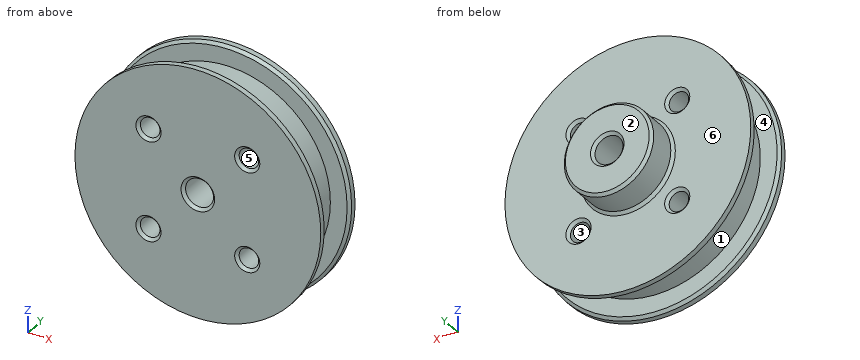
from build123d import *

# Parameters (mm, degrees)
F0_R      = 22
F1_DEPTH  = 5
F2_R      = 30.4296764291
F2_R_2    = 18.5
F3_DEPTH  = 3.5
F4_R      = 8
F5_DEPTH  = 6
F6_R      = 2.5
F7_DEPTH  = 16.001
F8_SIZE   = 0.5
F9_R      = 1.75
F10_DEPTH = 10.001
F11_SIZE  = 0.5


with BuildPart() as f1:
    # F0 (on Front) → F1 (new body, symmetric)
    with BuildSketch(Plane.XZ):
        Circle(F0_R)
    extrude(amount=F1_DEPTH, both=True)

    # F2 (on Front) → F3 (cut, symmetric)
    with BuildSketch(Plane.XZ):
        Circle(F2_R)
        Circle(F2_R_2, mode=Mode.SUBTRACT)
    extrude(amount=F3_DEPTH, both=True, mode=Mode.SUBTRACT)

    # F4 (on face) → F5 (join)
    with BuildSketch(Plane(origin=(0, 5, 0), x_dir=(-1, 0, 0), z_dir=(0, 1, 0))):
        Circle(F4_R)
    extrude(amount=F5_DEPTH)

    # F6 (on face) → F7 (cut, through all)
    with BuildSketch(Plane(origin=(0, 11, 0), x_dir=(-1, 0, 0), z_dir=(0, 1, 0))):
        Circle(F6_R)
    extrude(amount=-F7_DEPTH, mode=Mode.SUBTRACT)

    # F8
    f8_edges = [f1.edges().sort_by_distance(p)[0] for p in [
        (8, 11, 0),
        (2.5, 11, 0),
        (8, 5, 0),
        (-22, 3.5, 0),
        (-22, -3.5, 0),
        (2.5, -5, 0),
    ]]
    chamfer(f8_edges, length=F8_SIZE)

    # F9 (on face) → F10 (cut, through all)
    with BuildSketch(Plane(origin=(0, 5, 0), x_dir=(-1, 0, 0), z_dir=(0, 1, 0))):
        with Locations((-8.8388347648, 8.8388347648)):
            Circle(F9_R)
        with Locations((-8.8388347648, -8.8388347648)):
            Circle(F9_R)
        with Locations((8.8388347648, -8.8388347648)):
            Circle(F9_R)
        with Locations((8.8388347648, 8.8388347648)):
            Circle(F9_R)
    extrude(amount=-F10_DEPTH, mode=Mode.SUBTRACT)

    # F11
    f11_edges = [f1.edges().sort_by_distance(p)[0] for p in [
        (-7.088835, -5, 8.838835),
        (-7.088835, -5, -8.838835),
        (10.588835, -5, -8.838835),
        (10.588835, -5, 8.838835),
        (10.588835, 5, 8.838835),
        (-7.088835, 5, 8.838835),
        (-7.088835, 5, -8.838835),
        (10.588835, 5, -8.838835),
    ]]
    chamfer(f11_edges, length=F11_SIZE)


solid = f1.part
Design review of the part built by this model. Coordinates are the model's own, in mm. Face numbers are marked on the shaded views. A direction names the side the tool comes from. Coordinates: 2 decimals unless noted, no trailing zeros. Loops run counter-clockwise (first coordinate to the right, second up) from the corner with the lowest first, then second, coordinate; pieces in that order, holes last. Notation, with made-up numbers: M 20,-1 L 33,-1 A17 ccw 33,20 Z; hole C 17.25,9 d10. An arc over 180 degrees is marked long. Answer as CSV lines item,"result".
Item 1: Add section D-D on y = 8.5. State the section outline as (x, z) points, plus the area to 3 significant figures.
Answer list:
outline,"C 0,0 d16; hole C 0,0 d5"
area,"181 mm²"
Item 2: For P1, Ø6, axis at x = -1.5, y = 9, coming from the -Z side; P2, Ø5, axis at x = 12, y = 6, coming from the -Z side; P3, Ø1, axis at x = 16, y = 1, coming from the -Z side, all flat-tipped, find the tip position at first contact; note any pin that passes through.
Answer list:
P1,"z = -8"
P2,"z = -19.74"
P3,"z = -10.1"
Item 3: Add section C-C on y = 0.5. State the section outline as (x, z) points.
Answer list:
outline,"C 0,0 d37; hole C -8.84,-8.84 d3.5; hole C -8.84,8.84 d3.5; hole C 0,0 d5; hole C 8.84,-8.84 d3.5; hole C 8.84,8.84 d3.5"
Item 4: Machinability: for the marked faces 4, 5 and 6, which of the approach directions +Z, -Z, +X, -X, +Y, -Y give a long, thin tool a straight path to every point of the face, cutting with its end or side? Answer none if there is none.
Answer list:
face 4,"none"
face 5,"+Y, -Y"
face 6,"+Y"
Item 5: For probe 1 along Y at (x, z) = (-17.5, -10); probe 2 along Z at (x, y) = (0, 8.25); probe 3 along Z at (x, y) = (9, 3.25), list the stretches that pass through material, from the lowest coordinate up.
Answer list:
probe 1,"-5 to -3.5, 3.5 to 5"
probe 2,"-8 to -2.5, 2.5 to 8"
probe 3,"-16.16 to -10.58, -7.1 to 7.1, 10.58 to 16.16"
Item 6: The part is to be moulded in two halves that separate along X. For the marked faces 1, 2 and 3, say which applies: pulls with the +X half, pulls with the -X half, needs draft (parallel to the pull), parting line crosses it, or undercut.
Answer list:
face 1,"parting line crosses it"
face 2,"needs draft"
face 3,"undercut"
